Design review of the part built by this model. Coordinates are the model's own, in mm. Face numbers are marked on the shaded views. A direction names the side the tool comes from. Coordinates: 2 decimals unless noted, no trailing zeros. Write each loop counter-clockwise with the first axis right and the second up, starting at its lowest first coordinate (ties: lowest second). Pieces come first, ordered by that corner, then holes.
Q1. Add section A-A, the plane x = -47. Give the boundary of the cut face in (y, z).
Q2. The part is to be moulded in two halves that separate along X. For the marked faces 1, 2, 3 and 4, say which applies: +X half, -X half, draft (parallel to the pull), parting line (faces both ways), or undercut.
Q3. Add section C-C, the plane y = 41. Give the boundary of the cut face in (x, z), plus the area to 3 significant figures.
Q4. Add section D-D, the plane y = 94. Give the boundary of the cut face in (x, z), plus the area to 4 significant figures.
Q5. Add section B-B, the plane z = -10. Give the boundary of the cut face in (x, y), plus the area to 3 significant figures.
Q6. To check wall thickness, follow probe 1 along X at (y, z) = (148.5, -28.5); probe 2 along Y at (x, z) = (22.5, 21); probe 3 along Z at (x, y) = (75.8, 93). State the ranges of each line that lie inside material, in increasing order.
Q7. Machinability: for the marked faces 5 and 6, which of the approach directions +Z, -Z, +X, -X, +Y, -Y give a long, thin tool a straight path to every point of the face, cutting with its end or side? Answer none if there is none.
Q8. Clearance check with flat-ended pins moving along their axes: pin 1 Ø9.5 at (x, z) = (-47, -90) entering from -Y; pin 2 Ø10 at (x, z) = (-45, 69) entering from +Y; pin 3 Ø2 at (y, z) = (-1.5, 59) entering from +X; pin 4 Ø4 at (y, z) = (5.5, 53) entering from +X. State where each tip first meets the part, or that it passes through.
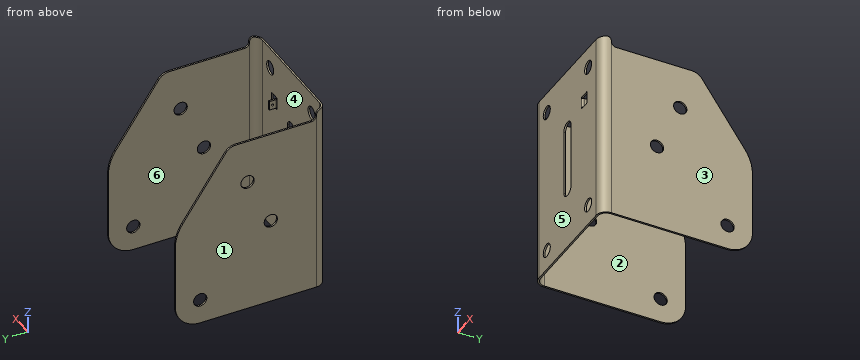
from build123d import *

# Parameters (mm, degrees)
SKETCH1_W                      = 150
SKETCH1_H                      = 230
BASE_FLANGE1_DEPTH             = 2
EDGE_FLANGE1_STRIP_W           = 28
EDGE_FLANGE1_STRIP_H           = 2
EDGE_FLANGE1_STRIP_CUT_DEPTH   = 230
EDGE_FLANGE1_STRIP_2_W         = 28
EDGE_FLANGE1_STRIP_2_H         = 2
EDGE_FLANGE1_STRIP_CUT_2_DEPTH = 230
EDGE_FLANGE1_DEPTH             = 230
EDGE_FLANGE1_BEND_DEPTH        = 230
SKETCH15_OUTSIDE_W             = 298.254
SKETCH15_OUTSIDE_H             = 250.254
SKETCH15_OUTSIDE_R             = 8
CUT_EXTRUDE1_DEPTH             = 264.326793168
SKETCH16_R                     = 8
CUT_EXTRUDE2_DEPTH             = 228.055059487
CUT_EXTRUDE3_DEPTH             = 228.055059487
SKETCHED_START                 = 47
SKETCHED_BEND1_DEPTH           = 11.052994728
SKETCHED_BEND1_2_DEPTH         = 11.052994728
CUT_EXTRUDE4_REACH             = 241.866
SKETCH20_R                     = 1.25


# Read off the part's stored shape, not the designer's step: Sketched Bend1
# Sheet-metal steps are written as plain solids
with BuildPart() as part:
    # Sketch1 → Base-Flange1 (new body)
    with BuildSketch(Plane(origin=(0, 0, 0), x_dir=(1, 0, 0), z_dir=(0, 1, 0))):
        Rectangle(SKETCH1_W, SKETCH1_H)
    extrude(amount=-BASE_FLANGE1_DEPTH)

    # Edge-Flange1 strip (across the edge) → Edge-Flange1 strip cut (cut)
    with BuildSketch(Plane(origin=(75, 0, 115), x_dir=(-1, 0, 0), z_dir=(0, 0, -1))):
        with Locations((-4, -1)):
            Rectangle(EDGE_FLANGE1_STRIP_W, EDGE_FLANGE1_STRIP_H)
    extrude(amount=EDGE_FLANGE1_STRIP_CUT_DEPTH, mode=Mode.SUBTRACT)

    # Edge-Flange1 strip 2 (across the edge) → Edge-Flange1 strip cut 2 (cut)
    with BuildSketch(Plane(origin=(-75, 0, -115), x_dir=(1, 0, 0), z_dir=(0, 0, 1))):
        with Locations((-4, -1)):
            Rectangle(EDGE_FLANGE1_STRIP_2_W, EDGE_FLANGE1_STRIP_2_H)
    extrude(amount=EDGE_FLANGE1_STRIP_CUT_2_DEPTH, mode=Mode.SUBTRACT)

    # Edge-Flange1 section (across the edge) → Edge-Flange1 (add)
    with BuildSketch(Plane(origin=(75, 0, 115), x_dir=(-1, 0, 0), z_dir=(0, 0, -1))):
        with BuildLine():
            Line((-2, 10), (-2, 180))
            Line((-2, 180), (0, 180))
            Line((0, 180), (0, 10))
            ThreePointArc((0, 10), (2.928932188, 2.928932188), (10, 0))
            Line((10, 0), (10, -2))
            ThreePointArc((10, -2), (1.514718626, 1.514718626), (-2, 10))
        make_face()
    extrude(amount=EDGE_FLANGE1_DEPTH)

    # Edge-Flange1 section 2 (across the edge) → Edge-Flange1 bend (add)
    with BuildSketch(Plane(origin=(-75, 0, -115), x_dir=(1, 0, 0), z_dir=(0, 0, 1))):
        with BuildLine():
            Line((-2, 10), (-2, 180))
            Line((-2, 180), (0, 180))
            Line((0, 180), (0, 10))
            ThreePointArc((0, 10), (2.928932188, 2.928932188), (10, 0))
            Line((10, 0), (10, -2))
            ThreePointArc((10, -2), (1.514718626, 1.514718626), (-2, 10))
        make_face()
    extrude(amount=EDGE_FLANGE1_BEND_DEPTH)

    # Sketch15 outside → Cut-Extrude1 (cut, through all)
    # profile 1 of 4: a face of its own
    with BuildSketch(Plane.ZY.offset(77)):
        with Locations((0, 89)):
            Rectangle(SKETCH15_OUTSIDE_W, SKETCH15_OUTSIDE_H)
        with BuildLine():
            Line((21.083470393, 171.180744276), (96.507242037, 119.243178795))
            ThreePointArc((96.507242037, 119.243178795), (101.277963521, 113.867184852), (103, 106.888955512))
            Line((103, 106.888955512), (103, 16))
            ThreePointArc((103, 16), (104.757359313, 11.757359313), (109, 10))
            Line((109, 10), (110, 10))
            ThreePointArc((110, 10), (113.535533906, 8.535533906), (115, 5))
            Line((115, 5), (115, -2))
            Line((115, -2), (-115, -2))
            Line((-115, -2), (-115, 99))
            Line((-115, 99), (-115, 150))
            ThreePointArc((-115, 150), (-106.213203436, 171.213203436), (-85, 180))
            Line((-85, 180), (-49, 180))
            Line((-49, 180), (-7.274003064, 180))
            ThreePointArc((-7.274003064, 180), (7.574612801, 177.744304445), (21.083470393, 171.180744276))
        make_face(mode=Mode.SUBTRACT)
    # profile 2 of 4: a face of its own
    with BuildSketch(Plane.ZY.offset(77)):
        with Locations(Location((50, 93, 0), (0, 0, 270))):
            Circle(SKETCH15_OUTSIDE_R)
    # profile 3 of 4: a face of its own
    with BuildSketch(Plane.ZY.offset(77)):
        with Locations(Location((-85, 150, 0), (0, 0, 270))):
            Circle(SKETCH15_OUTSIDE_R)
    # profile 4 of 4: a face of its own
    with BuildSketch(Plane.ZY.offset(77)):
        with Locations(Location((-10, 65, 0), (0, 0, 270))):
            Circle(SKETCH15_OUTSIDE_R)
    extrude(amount=-CUT_EXTRUDE1_DEPTH, mode=Mode.SUBTRACT)

    # Sketch16 → Cut-Extrude2 (cut, through all)
    with BuildSketch(Plane(origin=(0, 0, 0), x_dir=(1, 0, 0), z_dir=(0, 1, 0))):
        with Locations(Location((-47, 90, 0), (0, 0, 270))):
            Circle(SKETCH16_R)
        with Locations(Location((47, 90, 0), (0, 0, 90))):
            Circle(SKETCH16_R)
        with Locations(Location((47, -90, 0), (0, 0, 270))):
            Circle(SKETCH16_R)
        with Locations(Location((-47, -90, 0), (0, 0, 90))):
            Circle(SKETCH16_R)
        with BuildLine():
            Line((8, 40), (8, -40))
            ThreePointArc((8, -40), (0, -48), (-8, -40))
            Line((-8, -40), (-8, 40))
            ThreePointArc((-8, 40), (0, 48), (8, 40))
        make_face()
    extrude(amount=-CUT_EXTRUDE2_DEPTH, mode=Mode.SUBTRACT)

    # Sketch18 → Cut-Extrude3 (cut, through all)
    with BuildSketch(Plane(origin=(0, 0, 0), x_dir=(1, 0, 0), z_dir=(0, 1, 0))):
        Polygon((31.4, -45), (44.4, -45), (44.4, -60.052994728), (31.4, -60.052994728), (31.4, -58.052994728), (42.4, -58.052994728), (42.4, -47), (31.4, -47), align=None)
    extrude(amount=-CUT_EXTRUDE3_DEPTH, mode=Mode.SUBTRACT)

    # Sketched Bend1 outline → Sketched Bend1 (cut)
    with BuildSketch(Plane.XY.offset(SKETCHED_START)):
        with BuildLine():
            ThreePointArc((34.035602398, 0), (33.054267209, -1.443395312), (31.4, -2))
            Line((31.4, -2), (42.4, -2))
            Line((42.4, -2), (42.4, 0))
            Line((42.4, 0), (34.035602398, 0))
        make_face()
    extrude(amount=SKETCHED_BEND1_DEPTH, mode=Mode.SUBTRACT)

    # Sketched Bend1 2 outline → Sketched Bend1 2 (add)
    with BuildSketch(Plane.XY.offset(SKETCHED_START)):
        with BuildLine():
            Line((31.4, 0), (34.035602398, 0))
            ThreePointArc((34.035602398, 0), (34.111233029, 0.364854094), (34.1366, 0.7366))
            Line((34.1366, 0.7366), (34.1366, 9.008755099))
            Line((34.1366, 9.008755099), (32.1366, 9.008755099))
            Line((32.1366, 9.008755099), (32.1366, 0.7366))
            ThreePointArc((32.1366, 0.7366), (31.920854855, 0.215745145), (31.4, 0))
        make_face()
    extrude(amount=SKETCHED_BEND1_2_DEPTH)

    # Sketch20 → Cut-Extrude4 (cut, up to next)
    with BuildSketch(Plane.ZY.offset(-32.1366), mode=Mode.PRIVATE) as cut_extrude4_sk1:
        with Locations(Location((52.526497364, 4.9366, 0), (0, 0, 270))):
            Circle(SKETCH20_R)
    cut_extrude4_tool1 = extrude(cut_extrude4_sk1.sketch, amount=-CUT_EXTRUDE4_REACH, mode=Mode.PRIVATE) & part.part
    add(cut_extrude4_tool1.solids().sort_by_distance((32.1366, 4.9366, 52.526497))[0], mode=Mode.SUBTRACT)


solid = part.part
Here are the results:
1. outline: (-2, -115) - (0, -115) - (0, -98) - (-2, -98) - close; (-2, -82) - (0, -82) - (0, 82) - (-2, 82) - close; (-2, 98) - (0, 98) - (0, 115) - (-2, 115) - close
2. face 1: -X half
2. face 2: undercut
2. face 3: +X half
2. face 4: undercut
3. outline: (-77, -115) - (-75, -115) - (-75, 103) - (-77, 103) - close; (75, -115) - (77, -115) - (77, 103) - (75, 103) - close
3. area: 872 mm2
4. outline: (-77, -115) - (-75, -115) - (-75, 42.06) - (-77, 42.06) - close; (-77, 57.94) - (-75, 57.94) - (-75, 103) - (-77, 103) - close; (75, -115) - (77, -115) - (77, 42.06) - (75, 42.06) - close; (75, 57.94) - (77, 57.94) - (77, 103) - (75, 103) - close
4. area: 808.5 mm2
5. outline: (-77, 10) arc R12 ccw to (-65, -2) - (-8, -2) - (-8, 0) - (-65, 0) arc R10 cw to (-75, 10) - (-75, 57) - (-77, 57) - close; (-77, 73) - (-75, 73) - (-75, 180) - (-77, 180) - close; (8, -2) - (65, -2) arc R12 ccw to (77, 10) - (77, 57) - (75, 57) - (75, 10) arc R10 cw to (65, 0) - (8, 0) - close; (75, 73) - (77, 73) - (77, 180) - (75, 180) - close
5. area: 913 mm2
6. probe 1: x = -77 to -75, 75 to 77
6. probe 2: y = -2 to 0
6. probe 3: z = -115 to 42, 58 to 103
7. face 5: +Z, -Z, +X, -X, -Y
7. face 6: +Z, -Z, +Y
8. pin 1: passes through
8. pin 2: stops at y = 0
8. pin 3: stops at x = 70.81
8. pin 4: stops at x = 76.74
